Print and shaded views of the part. All mm, measured from the part's lowest x, y and z. Round coordinates to 2 decimals unless told otherwise and drop trailing zeros. Write each loop counter-clockwise with the first axis right and the second up, starting at its lowest first coordinate (ties: lowest second). Pieces come first, ordered by that corner, then holes. Notation, with made-up numbers: M 56.5,35.5 L 63.5,35.5 A33 cw 63.5,73.5 Z; hole C 86.25,30.5 d2. An arc over 180 degrees is marked long. Write item = value, one per line. Start each with the question number.
Q1. Drop a flat-ended pin along its axis: P1, Ø10, axis at x = 32.5, z = 17.5, coming from the +Y side. Give the stop position or say it passes through.
Q2. Probe L1, parallel to X at y = 18, z = 16.25; L2, parallel to X at y = 26, z = 14.75; L3, parallel to Z at x = 32, y = 3. List the from-to ranges inside material, lowest first.
Q3. Band-saw the part on A-A on z = 16.25. Write the cut outline in (x, y).
Q4. Band-saw the part on B-B on x = 11.25. Write the cut outline in (y, z).
Q5. Band-saw the part on C-C on y = 18. Write the cut outline in (x, z), plus the area to 3 significant figures.
Q6. Band-saw the part on D-D on z = 13. Write the cut outline in (x, y).
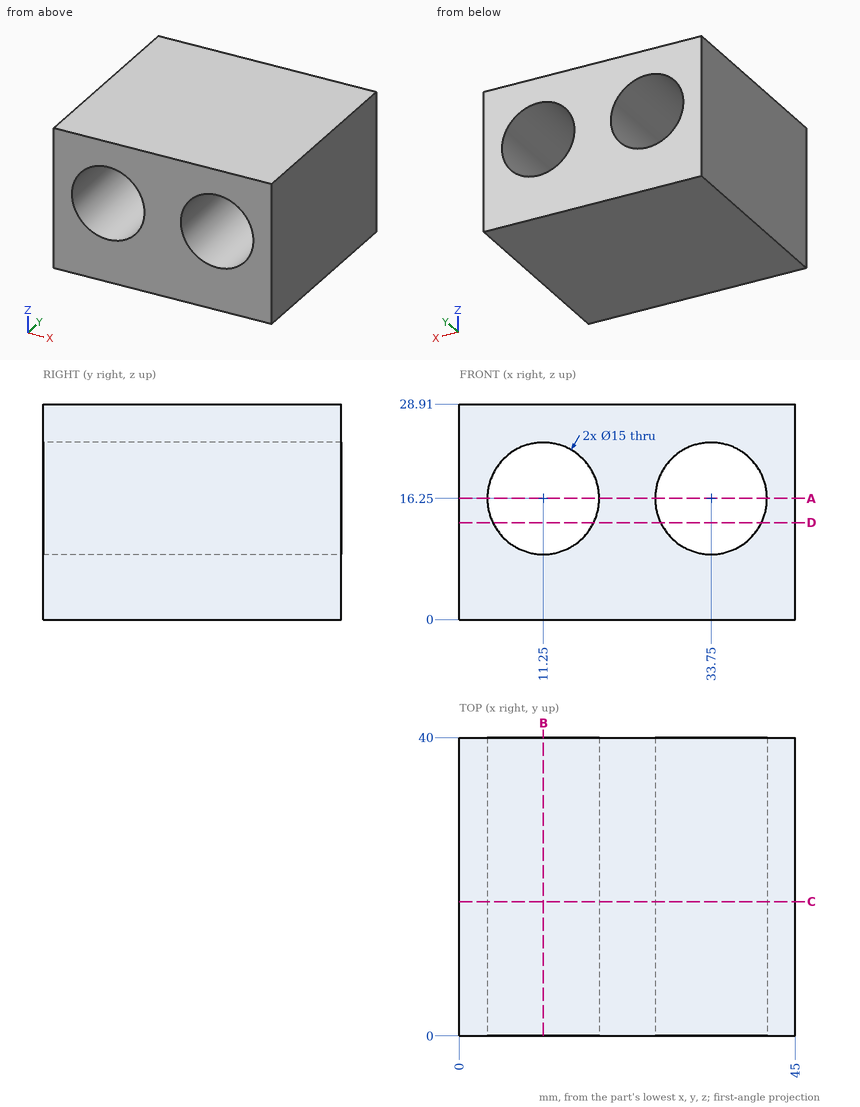
Conclusion:
q1.P1 = through
q2.L1 = 0 to 3.75, 18.75 to 26.25, 41.25 to 45
q2.L2 = 0 to 3.9, 18.6 to 26.4, 41.1 to 45
q2.L3 = 0 to 8.96, 23.54 to 28.91
q3.outline = M 0,0 L 3.75,0 L 3.75,40 L 0,40 Z; M 18.75,0 L 26.25,0 L 26.25,40 L 18.75,40 Z; M 41.25,0 L 45,0 L 45,40 L 41.25,40 Z
q4.outline = M 0,0 L 40,0 L 40,8.75 L 0,8.75 Z; M 0,23.75 L 40,23.75 L 40,28.91 L 0,28.91 Z
q5.outline = M 0,0 L 45,0 L 45,28.91 L 0,28.91 Z; hole C 11.25,16.25 d15; hole C 33.75,16.25 d15
q5.area = 948 mm^2
q6.outline = M 0,0 L 4.49,0 L 4.49,40 L 0,40 Z; M 18.01,0 L 26.99,0 L 26.99,40 L 18.01,40 Z; M 40.51,0 L 45,0 L 45,40 L 40.51,40 Z
